Work out the finished part from the listing and answer in its coordinate system (mm). A direction names the side the tool comes from. Coordinates: 2 decimals unless noted, no trailing zeros. Loops run counter-clockwise (first coordinate to the right, second up) from the corner with the lowest first, then second, coordinate; pieces in that order, holes last. Notation, with made-up numbers: (34, 19) - (72, 19) arc R23 cw to (72, 55) - close; hole circle Ø6 at (73.25, -28.5). An arc over 180 degrees is marked (long way). Write each question's results on one line, items separated by ' | '. Start each with the question number.
1. Find the intervals of material crossed by line 1 along Z through (x, y) = (12, 0); line 2 along X through (y, z) = (31, 5.5); line 3 along Z through (x, y) = (22, 0), in increasing order. Write a range as [from, to].
2. A cutting plane is placed at C-C on x = 12. Determine the outline of the cut face in (y, z), then the cut area to 3 significant figures.
3. Each of these flat-tipped pins is pushed along its axis until it touches: P1, Ø1, axis at x = 11, y = -16, coming from the +Z side; P2, Ø1, axis at x = 14.5, y = -23.5, coming from the +Z side; P3, Ø4, axis at x = 7, z = -26.5, coming from the +Y side. Where does it stop, or does it pass through?
4. Which of the six approach directions +Z, -Z, +X, -X, +Y, -Y give full straight-line access (tool end or side, diameter ignored) to faces 1 (the cylindrical face through (27.308, -13.887, -10.648)), 2 (the cylindrical face through (3.479, -4.686, 35.694)), 3 (the flat face through (35, -7, -7))?
5. A cutting plane is placed at A-A on y = 0. Determine the outline of the cut face in (x, z), then the cut area to 3 significant figures.
from build123d import *


with BuildPart() as part:
    # Sketch1 → Base-Revolve (revolve)
    with BuildSketch(Plane.XY):
        with BuildLine():
            Line((0, 9.5), (35, 9.5))
            Line((35, 9.5), (35, 16.5))
            Line((35, 16.5), (34, 17.5))
            Line((34, 17.5), (20.8, 17.5))
            ThreePointArc((20.8, 17.5), (20.234314575, 17.734314575), (20, 18.3))
            Line((20, 18.3), (20, 37))
            ThreePointArc((20, 37), (19.121320344, 39.121320344), (17, 40))
            Line((17, 40), (7.309401077, 40))
            Line((7.309401077, 40), (5, 36))
            Line((5, 36), (2, 36))
            Line((2, 36), (2, 35))
            Line((2, 35), (0, 35))
            Line((0, 35), (0, 9.5))
        make_face()
    revolve(axis=Axis((-31.276903974, 0, 0), (1, 0, 0)))


solid = part.part
Values:
1) line 1: [-40, -9.5], [9.5, 40] | line 2: [0, 20] | line 3: [-17.5, -9.5], [9.5, 17.5]
2) outline: circle Ø80 at (0, 0); hole circle Ø19 at (0, 0) | area: 4,740 mm^2
3) P1: z = 36.87 | P2: z = 32.73 | P3: y = 31.6
4) face 1: +X | face 2: -X | face 3: +Z, -Z, +X, +Y, -Y
5) outline: (0, -35) - (2, -35) - (2, -36) - (5, -36) - (7.31, -40) - (17, -40) arc R3 ccw to (20, -37) - (20, -18.3) arc R0.8 cw to (20.8, -17.5) - (34, -17.5) - (35, -16.5) - (35, -9.5) - (0, -9.5) - close; (0, 9.5) - (35, 9.5) - (35, 16.5) - (34, 17.5) - (20.8, 17.5) arc R0.8 cw to (20, 18.3) - (20, 37) arc R3 ccw to (17, 40) - (7.31, 40) - (5, 36) - (2, 36) - (2, 35) - (0, 35) - close | area: 1,400 mm^2
